```python
from build123d import *

# Parameters (mm, degrees)
SKETCH_1_R      = 1.6
SKETCH_1_R_2    = 1.5
EXTRUDE_1_DEPTH = 2


with BuildPart() as part:
    # 草图1 → 凸台-拉伸1 (new body)
    with BuildSketch(Plane.XY):
        with BuildLine():
            Line((-44.4, -52.5), (-48.4, -52.5))
            ThreePointArc((-48.4, -52.5), (-51.228427125, -53.671572875), (-52.4, -56.5))
            Line((-52.4, -56.5), (-52.4, -58.4))
            ThreePointArc((-52.4, -58.4), (-51.228427125, -61.228427125), (-48.4, -62.4))
            Line((-48.4, -62.4), (48.4, -62.4))
            ThreePointArc((48.4, -62.4), (51.228427125, -61.228427125), (52.4, -58.4))
            Line((52.4, -58.4), (52.4, 58.4))
            ThreePointArc((52.4, 58.4), (51.228427125, 61.228427125), (48.4, 62.4))
            Line((48.4, 62.4), (-48.4, 62.4))
            ThreePointArc((-48.4, 62.4), (-51.228427125, 61.228427125), (-52.4, 58.4))
            Line((-52.4, 58.4), (-52.4, 56.5))
            ThreePointArc((-52.4, 56.5), (-51.228427125, 53.671572875), (-48.4, 52.5))
            Line((-48.4, 52.5), (-44.4, 52.5))
            ThreePointArc((-44.4, 52.5), (-42.985786438, 51.914213562), (-42.4, 50.5))
            Line((-42.4, 50.5), (-42.4, 31.743164199))
            ThreePointArc((-42.4, 31.743164199), (-42.37587505, 31.433458229), (-42.304082212, 31.1312239))
            Line((-42.304082212, 31.1312239), (-34.476756551, 6.776116715))
            ThreePointArc((-34.476756551, 6.776116715), (-33.486356648, 5.608960434), (-31.96073404, 5.483974801))
            Line((-31.96073404, 5.483974801), (11.833156842, 19.558601667))
            ThreePointArc((11.833156842, 19.558601667), (13.35877945, 19.433616033), (14.349179353, 18.266459753))
            Line((14.349179353, 18.266459753), (22.304403233, -6.486609007))
            ThreePointArc((22.304403233, -6.486609007), (22.1794176, -8.012231615), (21.01226132, -9.002631517))
            Line((21.01226132, -9.002631517), (-16.278628995, -20.987302349))
            ThreePointArc((-16.278628995, -20.987302349), (-16.355786059, -21.010396022), (-16.433810344, -21.030364524))
            Line((-16.433810344, -21.030364524), (-26.148012146, -23.309111102))
            ThreePointArc((-26.148012146, -23.309111102), (-28.868282326, -25.00149387), (-30.002896471, -27.997604687))
            ThreePointArc((-30.002896471, -27.997604687), (-33.674500198, -32.259809436), (-38.636209823, -29.608677444))
            ThreePointArc((-38.636209823, -29.608677444), (-39.400357242, -28.365879544), (-40.490725679, -27.396568153))
            ThreePointArc((-40.490725679, -27.396568153), (-41.09539832, -27.234472424), (-41.677960491, -27.463656512))
            ThreePointArc((-41.677960491, -27.463656512), (-42.210513875, -28.15237372), (-42.4, -29.0021028))
            Line((-42.4, -29.0021028), (-42.4, -50.5))
            ThreePointArc((-42.4, -50.5), (-42.985786438, -51.914213562), (-44.4, -52.5))
        make_face()
        with Locations((-42.5, 57.5)):
            Circle(SKETCH_1_R, mode=Mode.SUBTRACT)
        with Locations((-23.596243703, 11.323307075)):
            Circle(SKETCH_1_R_2, mode=Mode.SUBTRACT)
        with Locations((-35, 35)):
            Circle(SKETCH_1_R_2, mode=Mode.SUBTRACT)
        with Locations((35, 35)):
            Circle(SKETCH_1_R_2, mode=Mode.SUBTRACT)
        with Locations((42.5, 57.5)):
            Circle(SKETCH_1_R, mode=Mode.SUBTRACT)
        with Locations((-42.5, -57.5)):
            Circle(SKETCH_1_R, mode=Mode.SUBTRACT)
        with Locations((42.5, -57.5)):
            Circle(SKETCH_1_R, mode=Mode.SUBTRACT)
        with Locations((35, -35)):
            Circle(SKETCH_1_R_2, mode=Mode.SUBTRACT)
        with Locations((-35, -35)):
            Circle(SKETCH_1_R_2, mode=Mode.SUBTRACT)
        with Locations((-12.58131833, -22.950172746)):
            Circle(SKETCH_1_R_2, mode=Mode.SUBTRACT)
        with Locations((20.978130661, -12.164724985)):
            Circle(SKETCH_1_R_2, mode=Mode.SUBTRACT)
        with Locations((9.963205288, 22.108754836)):
            Circle(SKETCH_1_R_2, mode=Mode.SUBTRACT)
        with BuildLine():
            Line((36.228402422, -50.292195812), (33.346068176, -39.754137802))
            ThreePointArc((33.346068176, -39.754137802), (32.661663143, -38.71633993), (31.496343748, -38.283367205))
            Line((31.496343748, -38.283367205), (-8.428369276, -36.696782686))
            ThreePointArc((-8.428369276, -36.696782686), (-10.482915991, -38.380786509), (-9.052823237, -40.619506186))
            Line((-9.052823237, -40.619506186), (33.754224033, -52.744148714))
            ThreePointArc((33.754224033, -52.744148714), (35.70708051, -52.240427548), (36.228402422, -50.292195812))
        make_face(mode=Mode.SUBTRACT)
        with BuildLine():
            Line((-11.169167715, -55.39772262), (14.676212639, -55.39772262))
            ThreePointArc((14.676212639, -55.39772262), (16.657197457, -53.672857401), (15.221250464, -51.473421768))
            Line((15.221250464, -51.473421768), (-22.734121612, -40.722964827))
            ThreePointArc((-22.734121612, -40.722964827), (-25.033361399, -41.686653646), (-24.606922294, -44.142941378))
            Line((-24.606922294, -44.142941378), (-12.496930572, -54.893398319))
            ThreePointArc((-12.496930572, -54.893398319), (-11.879325656, -55.267395238), (-11.169167715, -55.39772262))
        make_face(mode=Mode.SUBTRACT)
        with BuildLine():
            Line((-36.742590149, -55.165200028), (-22.049714315, -55.339653699))
            ThreePointArc((-22.049714315, -55.339653699), (-20.183876505, -54.118700422), (-20.607795776, -51.929552166))
            Line((-20.607795776, -51.929552166), (-31.792186791, -40.682261625))
            ThreePointArc((-31.792186791, -40.682261625), (-33.681632949, -40.148821509), (-35.116941327, -41.488394201))
            Line((-35.116941327, -41.488394201), (-38.625426146, -52.561231071))
            ThreePointArc((-38.625426146, -52.561231071), (-38.339555845, -54.337218436), (-36.742590149, -55.165200028))
        make_face(mode=Mode.SUBTRACT)
        with BuildLine():
            Line((-13.225378494, -25.687031503), (-20.97493997, -29.683652555))
            ThreePointArc((-20.97493997, -29.683652555), (-22.001813607, -31.932849454), (-20.05822519, -33.461188493))
            Line((-20.05822519, -33.461188493), (5.640197545, -33.461188493))
            ThreePointArc((5.640197545, -33.461188493), (7.628209121, -31.679843412), (6.074886055, -29.508998467))
            Line((6.074886055, -29.508998467), (-11.873975203, -25.512377414))
            ThreePointArc((-11.873975203, -25.512377414), (-12.565009854, -25.481063809), (-13.225378494, -25.687031503))
        make_face(mode=Mode.SUBTRACT)
        with BuildLine():
            Line((17.588533005, -15.747781939), (-1.043142169, -20.843855178))
            ThreePointArc((-1.043142169, -20.843855178), (-2.515026651, -22.816049848), (-0.959614951, -24.723060647))
            Line((-0.959614951, -24.723060647), (25.514222239, -30.752443796))
            ThreePointArc((25.514222239, -30.752443796), (27.619822805, -29.915706508), (27.593050924, -27.650101445))
            Line((27.593050924, -27.650101445), (19.750888908, -16.524645057))
            ThreePointArc((19.750888908, -16.524645057), (18.792402475, -15.794708381), (17.588533005, -15.747781939))
        make_face(mode=Mode.SUBTRACT)
        with BuildLine():
            Line((29.477837532, 7.795881804), (24.066416739, -11.309584207))
            ThreePointArc((24.066416739, -11.309584207), (24.010895626, -12.138003378), (24.296577485, -12.917584543))
            Line((24.296577485, -12.917584543), (29.707998278, -21.542258413))
            ThreePointArc((29.707998278, -21.542258413), (31.955184399, -22.401310498), (33.402138384, -20.479295902))
            Line((33.402138384, -20.479295902), (33.402138384, 7.250843979))
            ThreePointArc((33.402138384, 7.250843979), (31.677273166, 9.231828797), (29.477837532, 7.795881804))
        make_face(mode=Mode.SUBTRACT)
        with BuildLine():
            Line((24.026121987, 5.86217634), (30.248482278, 26.112145879))
            ThreePointArc((30.248482278, 26.112145879), (29.574516748, 28.270520689), (27.318372256, 28.420931424))
            Line((27.318372256, 28.420931424), (17.195320702, 22.43221936))
            ThreePointArc((17.195320702, 22.43221936), (16.359901321, 21.461624711), (16.284509384, 20.183229009))
            Line((16.284509384, 20.183229009), (20.185200647, 5.921971534))
            ThreePointArc((20.185200647, 5.921971534), (22.083209124, 4.4498659), (24.026121987, 5.86217634))
        make_face(mode=Mode.SUBTRACT)
        with BuildLine():
            Line((26.466941663, 32.346827687), (31.13344693, 34.889103877))
            ThreePointArc((31.13344693, 34.889103877), (31.67231487, 35.317620871), (32.033943195, 35.903479579))
            Line((32.033943195, 35.903479579), (34.005211961, 40.838410083))
            ThreePointArc((34.005211961, 40.838410083), (33.198419308, 43.282203141), (30.652232239, 42.908077088))
            Line((30.652232239, 42.908077088), (24.014458205, 35.430870394))
            ThreePointArc((24.014458205, 35.430870394), (23.944750718, 32.85828808), (26.466941663, 32.346827687))
        make_face(mode=Mode.SUBTRACT)
        with BuildLine():
            Line((12.639411879, 29.541355608), (28.719343057, 47.084579709))
            ThreePointArc((28.719343057, 47.084579709), (28.952178023, 49.477824874), (26.717325897, 50.365107531))
            Line((26.717325897, 50.365107531), (7.292247383, 45.052025274))
            ThreePointArc((7.292247383, 45.052025274), (6.082684716, 44.113886743), (5.89075887, 42.595232661))
            Line((5.89075887, 42.595232661), (9.235906205, 30.365090816))
            ThreePointArc((9.235906205, 30.365090816), (10.694578809, 28.948865324), (12.639411879, 29.541355608))
        make_face(mode=Mode.SUBTRACT)
        with BuildLine():
            Line((-6.119101541, 26.393542701), (-9.484773183, 36.865994869))
            ThreePointArc((-9.484773183, 36.865994869), (-10.475173086, 38.033151149), (-12.000795694, 38.158136783))
            Line((-12.000795694, 38.158136783), (-22.473247861, 34.792465141))
            ThreePointArc((-22.473247861, 34.792465141), (-23.640404142, 33.802065238), (-23.765389775, 32.27644263))
            Line((-23.765389775, 32.27644263), (-20.399718133, 21.803990463))
            ThreePointArc((-20.399718133, 21.803990463), (-19.40931823, 20.636834182), (-17.883695622, 20.511848549))
            Line((-17.883695622, 20.511848549), (-7.411243455, 23.877520191))
            ThreePointArc((-7.411243455, 23.877520191), (-6.244087174, 24.867920093), (-6.119101541, 26.393542701))
        make_face(mode=Mode.SUBTRACT)
        with BuildLine():
            Line((-21.208612958, 41.544719282), (12.954393861, 50.888870206))
            ThreePointArc((12.954393861, 50.888870206), (14.410493094, 53.072433346), (12.450486839, 54.817869808))
            Line((12.450486839, 54.817869808), (-9.100688804, 55.073754479))
            ThreePointArc((-9.100688804, 55.073754479), (-9.752383451, 54.972758068), (-10.335803304, 54.66530488))
            Line((-10.335803304, 54.66530488), (-22.947634479, 45.065269285))
            ThreePointArc((-22.947634479, 45.065269285), (-23.529428542, 42.588103366), (-21.208612958, 41.544719282))
        make_face(mode=Mode.SUBTRACT)
        with BuildLine():
            Line((-38.466382383, 52.758728631), (-35.036841892, 42.623668672))
            ThreePointArc((-35.036841892, 42.623668672), (-33.702415155, 41.344743502), (-31.889657598, 41.705651167))
            Line((-31.889657598, 41.705651167), (-19.509525421, 51.652997335))
            ThreePointArc((-19.509525421, 51.652997335), (-18.871772637, 53.864883905), (-20.738488051, 55.211934154))
            Line((-20.738488051, 55.211934154), (-36.548160719, 55.399647945))
            ThreePointArc((-36.548160719, 55.399647945), (-38.190090809, 54.57515145), (-38.466382383, 52.758728631))
        make_face(mode=Mode.SUBTRACT)
    extrude(amount=EXTRUDE_1_DEPTH)


solid = part.part
```
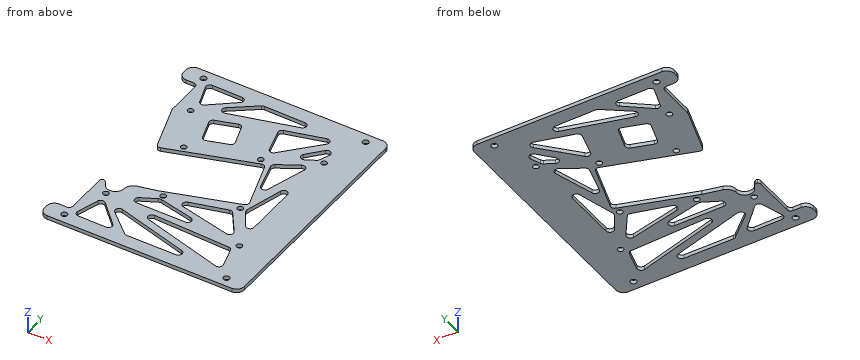
The listing builds one solid part. Answer for the finished solid, in the listing's coordinates (mm). Coordinates: 2 decimals unless noted, no trailing zeros. Write each loop counter-clockwise with the first axis right and the second up, starting at its lowest first coordinate (ties: lowest second). Pieces come first, ordered by that corner, then holes. Notation, with made-up numbers: (-32, -35.75) - (-21, -35.75) arc R24 cw to (-21, -22.75) - close; hole circle Ø3 at (9.5, -4.5). An arc over 180 degrees is marked (long way). Return JSON: item names as keys, results as strings. Group by question number.
Q1. Flat-ended cylindrical pins translate along their axes: pin 1 Ø0.6 at (y, z) = (-38, 0.5) entering from -X; pin 2 Ø1 at (y, z) = (-0.5, 0.5) entering from -X. Find the tip coordinate at first contact, or state that the pin passes through.
Q2. The part is cut by section A-A on y = -35. Write down the section's boundary in (x, z).
Q3. Find the intervals of material crossed by line 1 along Y through (x, z) = (-28, 1.15); line 2 along Y through (x, z) = (-27.5, 0.5); line 3 along X through (y, z) = (-33, 0.4), in increasing order. Write a range as [from, to].
Q4. The part is cut by section B-B on z = 0.8. State how many separate pieces and enclosed holes the cut face has, and give its area (3 significant figures).
Evaluation:
{
 "1": {"pin 1": "stops at x = -42.4", "pin 2": "stops at x = 20.22"},
 "2": {"outline": "(-42.4, 0) - (-36.5, 0) - (-36.5, 2) - (-42.4, 2) - close; (-33.5, 0) - (33.5, 0) - (33.5, 2) - (-33.5, 2) - close; (36.5, 0) - (52.4, 0) - (52.4, 2) - (36.5, 2) - close"},
 "3": {"line 1": "y = [-62.4, -55.27], [-44.5, -24.17], [6.76, 44.83], [55.3, 62.4]", "line 2": "y = [-62.4, -55.27], [-45, -23.84], [6.92, 45.23], [55.29, 62.4]", "line 3": "x = [-42.4, -21.34], [6.92, 52.4]"},
 "4": {"separate pieces": "1", "enclosed holes": "24", "area": "7,150 mm2"}
}
